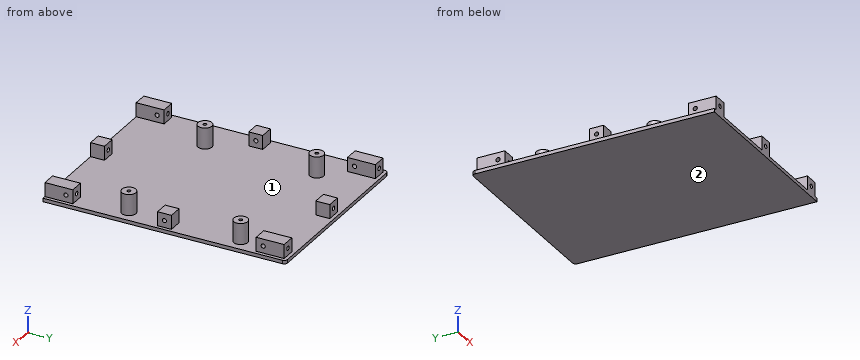
from build123d import *

# Parameters (mm, degrees)
F1_W      = 135
F1_H      = 173.65
F2_DEPTH  = 1.25
F3_W      = 10
F3_H      = 10
F3_H_2    = 20
F4_DEPTH  = 11.25
F5_R      = 5
F5_R_2    = 1.25
F6_DEPTH  = 16.25
F7_R      = 2.5
F16_D     = 3
F16_DEPTH = 25
F16_TIP   = 0.9012909285
F17_D     = 3
F17_DEPTH = 25
F17_TIP   = 0.9012909285
F18_D     = 3
F18_DEPTH = 25
F18_TIP   = 0.9012909285
F19_D     = 3
F19_DEPTH = 25
F19_TIP   = 0.9012909285


with BuildPart() as f2:
    # F1 (on offset) → F2 (new body, symmetric)
    with BuildSketch(Plane.XY.offset(-7.5)):
        with Locations((-1.75834e-05, 0.0049936295)):
            Rectangle(F1_W, F1_H)
    extrude(amount=F2_DEPTH, both=True)

    # F3 (on offset) → F4 (join)
    with BuildSketch(Plane.XY.offset(-7.5)):
        with Locations((-60.0000175834, -1.2700063705)):
            Rectangle(F3_W, F3_H)
        with Locations((-1.75834e-05, 79.3299936295)):
            Rectangle(F3_W, F3_H)
        with Locations((-60.0000175834, 74.3299936295)):
            Rectangle(F3_W, F3_H_2)
        with Locations((-60.0000175834, -76.8200063705)):
            Rectangle(F3_W, F3_H_2)
        with Locations((-1.75834e-05, -81.8200063705)):
            Rectangle(F3_W, F3_H)
        with Locations((60.0000175834, -1.2700063705)):
            Rectangle(F3_W, F3_H)
        with Locations((60.0000175834, 74.3299936295)):
            Rectangle(F3_W, F3_H_2)
        with Locations((60.0000175834, -76.8200063705)):
            Rectangle(F3_W, F3_H_2)
    extrude(amount=F4_DEPTH)

    # F5 (on offset) → F6 (join)
    with BuildSketch(Plane.XY.offset(-7.5)):
        with Locations((-42.5000175834, 49.1799936295)):
            Circle(F5_R)
        with Locations((-42.5000175834, 49.1799936295)):
            Circle(F5_R_2, mode=Mode.SUBTRACT)
        with Locations((-42.5000175834, -30.8200063705)):
            Circle(F5_R)
        with Locations((-42.5000175834, -30.8200063705)):
            Circle(F5_R_2, mode=Mode.SUBTRACT)
        with Locations((57.4999824166, -30.8200063705)):
            Circle(F5_R)
        with Locations((57.4999824166, -30.8200063705)):
            Circle(F5_R_2, mode=Mode.SUBTRACT)
        with Locations((57.4999824166, 49.1799936295)):
            Circle(F5_R)
        with Locations((57.4999824166, 49.1799936295)):
            Circle(F5_R_2, mode=Mode.SUBTRACT)
    extrude(amount=F6_DEPTH)

    # F7
    f7_edges = [f2.edges().sort_by_distance(p)[0] for p in [
        (-67.500018, 86.829994, -7.5),
        (67.499982, 86.829994, -7.5),
    ]]
    fillet(f7_edges, radius=F7_R)

    # F16
    with Locations(Plane.XZ.offset(88)):
        with Locations((-60.0000175834, -1.25), (0, -1.25), (59.9999824166, -1.25)):
            Hole(F16_D / 2, depth=F16_DEPTH)
            with Locations((0, 0, -(F16_DEPTH + F16_TIP / 2))):  # 118° drill point
                Cone(0, F16_D / 2, F16_TIP, mode=Mode.SUBTRACT)

    # F17
    with Locations(Plane.YZ.offset(70)):
        with Locations((-71.8200063705, -1.25), (-1.3229202013, -1.25), (69.3299936295, -1.25)):
            Hole(F17_D / 2, depth=F17_DEPTH)
            with Locations((0, 0, -(F17_DEPTH + F17_TIP / 2))):  # 118° drill point
                Cone(0, F17_D / 2, F17_TIP, mode=Mode.SUBTRACT)

    # F18
    with Locations(Plane(origin=(0, 90, 0), x_dir=(1, 0, 0), z_dir=(0, 1, 0))):
        with Locations((59.9999824166, 1.25), (0, 1.25), (-60.0000175834, 1.25)):
            Hole(F18_D / 2, depth=F18_DEPTH)
            with Locations((0, 0, -(F18_DEPTH + F18_TIP / 2))):  # 118° drill point
                Cone(0, F18_D / 2, F18_TIP, mode=Mode.SUBTRACT)

    # F19
    with Locations(Plane(origin=(-70.5, 0, 0), x_dir=(0, 1, 0), z_dir=(-1, 0, 0))):
        with Locations((69.3299936295, 1.30720163), (-1.2326835422, 1.25), (-71.8200063705, 1.25)):
            Hole(F19_D / 2, depth=F19_DEPTH)
            with Locations((0, 0, -(F19_DEPTH + F19_TIP / 2))):  # 118° drill point
                Cone(0, F19_D / 2, F19_TIP, mode=Mode.SUBTRACT)


solid = f2.part
Geometry check sheet. Reference: the model listing, model coordinates, mm. Face numbers are marked on the shaded views. Give positions to 0.01 mm unless a question says otherwise; leave off trailing zeros. Order: outer loops, then holes, each group sorted by start corner. A loop starts at its lowest first (then second) coordinate and runs counter-clockwise, first axis right, second up.
1) Gauge pin test, flat ends, axial feed: pin 1 (4 mm diameter, centred on x = 60, z = -1.25, fed in from +Y); pin 2 (5 mm diameter, centred on y = -4, z = 5, fed in from -X); pin 3 (2.5 mm diameter, centred on y = -71.82, z = -1.25, fed in from +X); pin 4 (8 mm diameter, centred on x = -62, z = -2.5, fed in from +Y). Record the tip position at first contact, or that the pin passes through.
Results are:
pin 1: stops at y = 84.33
pin 2: stops at x = -65
pin 3: passes through
pin 4: stops at y = 86.83
2) Cross-section at B-B (x = -35). Record the boundary of the cut face in (y, z).
Results are:
outline: (-86.82, -8.75) - (86.83, -8.75) - (86.83, -6.25) - (-86.82, -6.25) - close
3) Material ranges on probe 1 along Z at (x, y) = (-53, -67), recorded low to high.
Results are:
probe 1: z = -8.75 to -6.25
4) Cross-section at C-C (y = -11.5). Record the boundary of the cut face in (x, z), then the cut area to 4 significant figures.
Results are:
outline: (-67.5, -8.75) - (67.5, -8.75) - (67.5, -6.25) - (-67.5, -6.25) - close
area: 337.5 mm2
5) Draft check along X on the marked faces 1 and 2. Enter one of: released by +X, released by -X, zero draft, split by the parting line, or undercut.
Results are:
face 1: undercut
face 2: zero draft
6) Cross-section at A-A (z = 6.5). Record the boundary of the cut face in (x, y), then the cut area to 3 significant figures.
Results are:
outline: circle Ø10 at (-42.5, -30.82); circle Ø10 at (-42.5, 49.18); circle Ø10 at (57.5, -30.82); circle Ø10 at (57.5, 49.18); hole circle Ø2.5 at (-42.5, -30.82); hole circle Ø2.5 at (-42.5, 49.18); hole circle Ø2.5 at (57.5, -30.82); hole circle Ø2.5 at (57.5, 49.18)
area: 295 mm2
